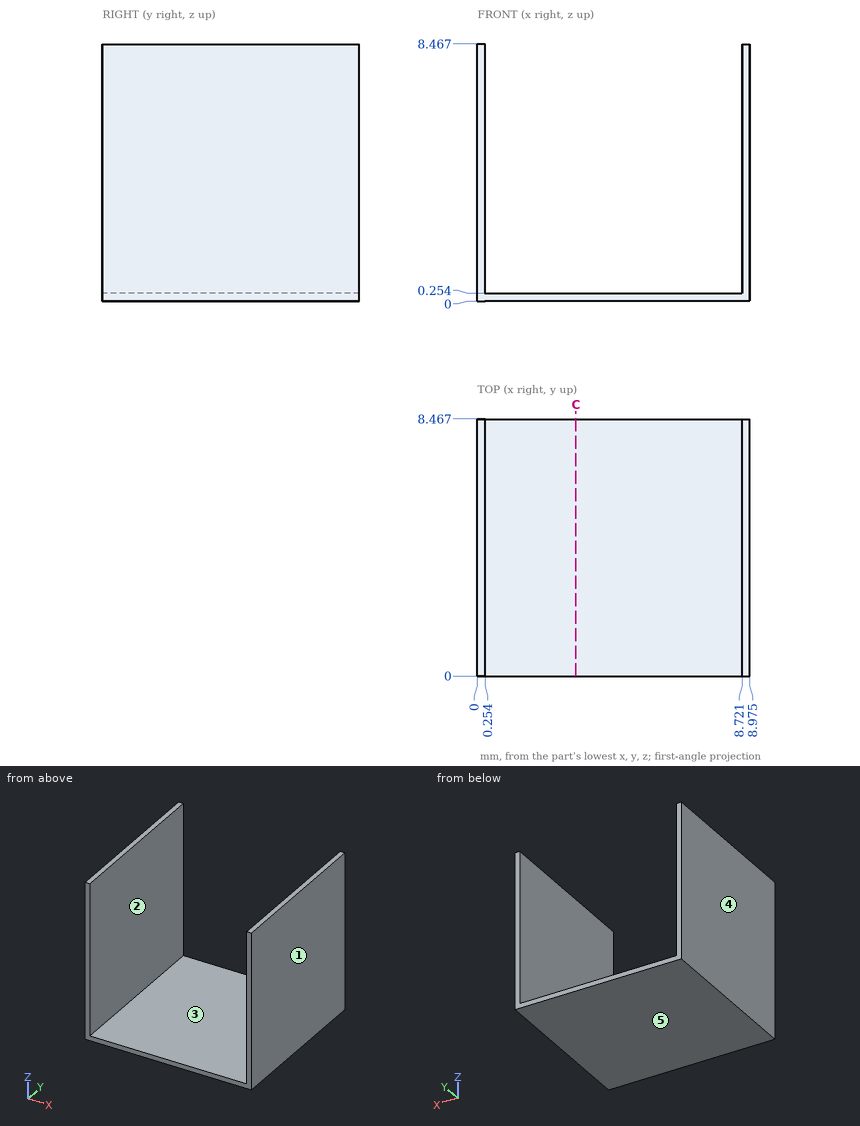
Part print with two shaded views. Sizes in mm from the minimum x, y, z corner. A direction names the side the tool comes from. Round coordinates to 2 decimals unless told otherwise and drop trailing zeros. Write each loop counter-clockwise with the first axis right and the second up, starting at its lowest first coordinate (ties: lowest second). Pieces come first, ordered by that corner, then holes. Notation, with made-up numbers: (43.5, 40) -> (91.5, 40) arc R22 cw to (91.5, 51) -> close; hole circle Ø9 at (8.5, -22.5). An arc over 180 degrees is marked (long way). Put each result on its own line as item: value.
Item 1: Slice it at C-C, the plane x = 3.25. Give the cut face in (y, z).
Here are the results:
outline: (0, 0) -> (8.47, 0) -> (8.47, 0.25) -> (0, 0.25) -> close
Item 2: Wall check: probe 1 along X at (y, z) = (3.75, 2.5) (1 decimal); probe 2 along Z at (x, y) = (1.25, 7.75). Give the ranges that are in metal, low to high. Write a range as from..to.
Here are the results:
probe 1: x = 0..0.3, 8.7..9
probe 2: z = 0..0.25
Item 3: Two-plate mould, pull along X, no slides. Class the marked faces 3, 4 and 5: pulls with the +X half, pulls with the -X half, needs draft (parallel to the pull), parting line crosses it, or undercut.
Here are the results:
face 3: undercut
face 4: pulls with the -X half
face 5: needs draft
Item 4: Flat gauge pins, fed straight in: P1, Ø1.5, axis at x = 6.5, y = 2.5, coming from the +Z side; P2, Ø2.5, axis at y = 4.5, z = 5, coming from the -X side. Where does each tip first touch, or does it go through?
Here are the results:
P1: stops at z = 0.25
P2: stops at x = 0
Item 5: Tool access for the marked faces 1 and 2: list every direction of +Z, -Z, +X, -X, +Y, -Y with a clear straight run to the whole face (end or side of a thin tool).
Here are the results:
face 1: +Z, -Z, +X, +Y, -Y
face 2: +Z, +Y, -Y
